Input: part model. Units: mm. Frame: model coordinates. Give positions to 0.01 mm unless a question says otherwise; leave off trailing zeros. Order: outer loops, then holes, each group sorted by start corner. A loop starts at its lowest first (then second) coordinate and runs counter-clockwise, first axis right, second up.
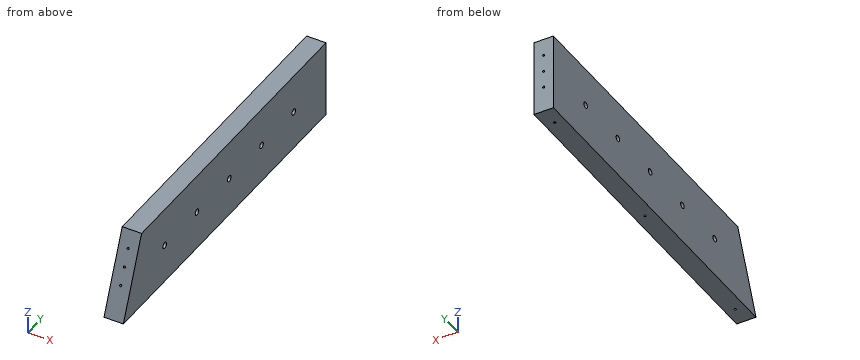
```python
from build123d import *

# Parameters (mm, degrees)
SKETCH1_W                            = 19.05
SKETCH1_H                            = 341.988103331
BOSS_EXTRUDE1_DEPTH                  = 76.2
CUT_EXTRUDE1_REACH                   = 21.05
F_5_64_0_07813_DIAMETER_HOLE1_D      = 1.984502
F_5_64_0_07813_DIAMETER_HOLE1_DEPTH  = 38.1
F_5_64_0_07813_DIAMETER_HOLE1_TIP    = 0.59620455
F_5_64_0_07813_DIAMETER_HOLE2_D      = 1.984502
F_5_64_0_07813_DIAMETER_HOLE2_DEPTH  = 38.1
F_5_64_0_07813_DIAMETER_HOLE2_TIP    = 0.59620455
F_5_64_0_07813_DIAMETER_HOLE3_D      = 1.984502
F_5_64_0_07813_DIAMETER_HOLE3_DEPTH  = 19.05
F_5_64_0_07813_DIAMETER_HOLE3_TIP    = 0.59620455
F_5_64_0_07813_DIAMETER_HOLE4_D      = 1.984502
F_5_64_0_07813_DIAMETER_HOLE4_DEPTH  = 19.05
F_5_64_0_07813_DIAMETER_HOLE4_TIP    = 0.59620455
F_15_64_0_23438_DIAMETER_HOLE1_D     = 5.953252
F_15_64_0_23438_DIAMETER_HOLE1_DEPTH = 19.05


with BuildPart() as part:
    # Sketch1 → Boss-Extrude1 (new body)
    with BuildSketch(Plane.XY):
        with Locations((485.002307398, 6812.735938475)):
            Rectangle(SKETCH1_W, SKETCH1_H)
    extrude(amount=BOSS_EXTRUDE1_DEPTH)

    # Sketch2 → Cut-Extrude1 (cut, up to next)
    with BuildSketch(Plane(origin=(494.527307398, 0, 0), x_dir=(0, 0, -1), z_dir=(1, 0, 0)), mode=Mode.PRIVATE) as cut_extrude1_sk1:
        Polygon((0, 6641.741886809), (-76.2, 6672.528685257), (-76.2, 6641.741886809), align=None)
    cut_extrude1_tool1 = extrude(cut_extrude1_sk1.sketch, amount=-CUT_EXTRUDE1_REACH, mode=Mode.PRIVATE) & part.part
    add(cut_extrude1_tool1.solids().sort_by_distance((494.527307, 6652.004153, 50.8))[0], mode=Mode.SUBTRACT)

    # 5/64 (0.07813) Diameter Hole1
    with Locations(Plane(origin=(0, -8e-09, -19.049996974), x_dir=(-1, 0, 0), z_dir=(0, 0, -1))):
        with Locations((-481.589248274, 6993.254992531), (-386.339248274, 6993.254992531), (-291.089248274, 6993.254992531), (-295.274999999, 6965.135938475), (-295.274999999, 6812.735938475), (-295.274999999, 6660.335938474), (-285.166362357, 6631.468843414), (-475.477307398, 6631.468752771), (-485.002307398, 6660.335938474), (-485.002307398, 6812.735938474), (-485.002307398, 6965.135938474), (-478.365617646, 6611.6708), (-287.865617646, 6611.6708), (-307.975, 6564.3379), (-307.975, 6488.1379), (-284.960913066, 6440.805), (-380.210913066, 6440.805), (-475.460913066, 6440.805), (-446.831312422, 6488.1379), (-446.831312422, 6564.3379), (-472.231312422, 6396.355), (-472.231312422, 6320.155), (-472.653156211, 6275.705000839), (-377.403156211, 6275.705000839), (-282.153156211, 6275.705000839), (-282.575, 6320.155), (-282.575, 6396.355), (-435.598646187, 6221.729999816), (-435.598646187, 6145.529999816), (-450.592518112, 6091.554999951), (-460.998646187, 6091.555478285), (-460.998646187, 6056.629999944), (-460.998646187, 5980.429999944), (-460.998646187, 5945.505000042), (-282.153156211, 5945.505000042), (-368.611823093, 5945.505000042)):
            Hole(F_5_64_0_07813_DIAMETER_HOLE1_D / 2, depth=F_5_64_0_07813_DIAMETER_HOLE1_DEPTH)
            with Locations((0, 0, -(F_5_64_0_07813_DIAMETER_HOLE1_DEPTH + F_5_64_0_07813_DIAMETER_HOLE1_TIP / 2))):  # 118° drill point
                Cone(0, F_5_64_0_07813_DIAMETER_HOLE1_D / 2, F_5_64_0_07813_DIAMETER_HOLE1_TIP, mode=Mode.SUBTRACT)

    # 5/64 (0.07813) Diameter Hole2
    with Locations(Plane(origin=(189.727307399, 0, -19.050000054), x_dir=(-1, 0, 0), z_dir=(0, 0, -1))):
        with Locations((-481.589248274, 6993.254992531), (-386.339248274, 6993.254992531), (-291.089248274, 6993.254992531), (-295.274999999, 6965.135938475), (-295.274999999, 6812.735938475), (-295.274999999, 6660.335938474), (-285.166362357, 6631.468843414), (-475.477307398, 6631.468752771), (-485.002307398, 6660.335938474), (-485.002307398, 6812.735938474), (-485.002307398, 6965.135938474), (-478.365617646, 6611.6708), (-287.865617646, 6611.6708), (-307.975, 6564.3379), (-307.975, 6488.1379), (-284.960913066, 6440.805), (-380.210913066, 6440.805), (-475.460913066, 6440.805), (-446.831312422, 6488.1379), (-446.831312422, 6564.3379), (-472.231312422, 6396.355), (-472.231312422, 6320.155), (-472.653156211, 6275.705000839), (-377.403156211, 6275.705000839), (-282.153156211, 6275.705000839), (-282.575, 6320.155), (-282.575, 6396.355), (-435.598646187, 6221.729999816), (-435.598646187, 6145.529999816), (-450.592518112, 6091.554999951), (-460.998646187, 6091.555478285), (-460.998646187, 6056.629999944), (-460.998646187, 5980.429999944), (-460.998646187, 5945.505000042), (-282.153156211, 5945.505000042), (-368.611823093, 5945.505000042)):
            Hole(F_5_64_0_07813_DIAMETER_HOLE2_D / 2, depth=F_5_64_0_07813_DIAMETER_HOLE2_DEPTH)
            with Locations((0, 0, -(F_5_64_0_07813_DIAMETER_HOLE2_DEPTH + F_5_64_0_07813_DIAMETER_HOLE2_TIP / 2))):  # 118° drill point
                Cone(0, F_5_64_0_07813_DIAMETER_HOLE2_D / 2, F_5_64_0_07813_DIAMETER_HOLE2_TIP, mode=Mode.SUBTRACT)

    # 5/64 (0.07813) Diameter Hole3
    with Locations(Plane(origin=(-4e-09, 6983.72999014, 0), x_dir=(1, 0, 0), z_dir=(0, 1, 0))):
        with Locations((485.002307402, -59.266666667), (485.002307402, -25.4), (485.002307402, -42.333333333)):
            Hole(F_5_64_0_07813_DIAMETER_HOLE3_D / 2, depth=F_5_64_0_07813_DIAMETER_HOLE3_DEPTH)
            with Locations((0, 0, -(F_5_64_0_07813_DIAMETER_HOLE3_DEPTH + F_5_64_0_07813_DIAMETER_HOLE3_TIP / 2))):  # 118° drill point
                Cone(0, F_5_64_0_07813_DIAMETER_HOLE3_D / 2, F_5_64_0_07813_DIAMETER_HOLE3_TIP, mode=Mode.SUBTRACT)

    # 5/64 (0.07813) Diameter Hole4
    with Locations(Plane(origin=(0, 5709.705582748, -2306.870800158), x_dir=(-1, 0, 0), z_dir=(0, -0.927183854, 0.374606594))):
        with Locations((-485.002307398, -2519.790305282), (-485.002307398, -2553.413203553), (-485.002307398, -2536.601754417)):
            Hole(F_5_64_0_07813_DIAMETER_HOLE4_D / 2, depth=F_5_64_0_07813_DIAMETER_HOLE4_DEPTH)
            with Locations((0, 0, -(F_5_64_0_07813_DIAMETER_HOLE4_DEPTH + F_5_64_0_07813_DIAMETER_HOLE4_TIP / 2))):  # 118° drill point
                Cone(0, F_5_64_0_07813_DIAMETER_HOLE4_D / 2, F_5_64_0_07813_DIAMETER_HOLE4_TIP, mode=Mode.SUBTRACT)

    # 15/64 (0.23438) Diameter Hole1
    with Locations(Plane.ZY.offset(-475.477307398)):
        with Locations((38.1, 6711.567736717), (38.1, 6929.297539455), (38.1, 6874.865088771), (38.1, 6820.432638086), (38.1, 6766.000187402)):
            Hole(F_15_64_0_23438_DIAMETER_HOLE1_D / 2, depth=F_15_64_0_23438_DIAMETER_HOLE1_DEPTH)


solid = part.part
```
1) First-contact query: P1, Ø2, axis at x = 489, z = 11, coming from the -Y side; P2, Ø1.8, axis at x = 485, y = 6660.34, coming from the +Z side; P3, Ø1.8, axis at x = 485, z = 42.33, coming from the -Y side. Flat tips, straight axial feed; report the tip coordinate or a pass-through.
2) Cut plane A-A (x = 478.75). Return the cut outline in (y, z).
3) Line query: probe 1 along Y at (x, z) = (492.75, 40.5); probe 2 along Z at (x, y) = (490, 6712); probe 3 along Y at (x, z) = (479.5, 38). Output: solid intervals per line, ascending.
Geometry says:
1. P1: stops at y = 6645.78
1. P2: stops at z = 48.26
1. P3: stops at y = 6658.48
2. outline: (6641.74, 0) - (6983.73, 0) - (6983.73, 76.2) - (6672.53, 76.2) - close; hole circle Ø5.95 at (6711.57, 38.1); hole circle Ø5.95 at (6766, 38.1); hole circle Ø5.95 at (6820.43, 38.1); hole circle Ø5.95 at (6874.87, 38.1); hole circle Ø5.95 at (6929.3, 38.1)
3. probe 1: y = 6658.1 to 6709.81, 6713.33 to 6764.24, 6767.76 to 6818.67, 6822.19 to 6873.1, 6876.63 to 6927.54, 6931.06 to 6983.73
3. probe 2: z = 0 to 35.15, 41.05 to 76.2
3. probe 3: y = 6657.09 to 6708.59, 6714.54 to 6763.03, 6768.98 to 6817.46, 6823.41 to 6871.89, 6877.84 to 6926.32, 6932.27 to 6983.73
